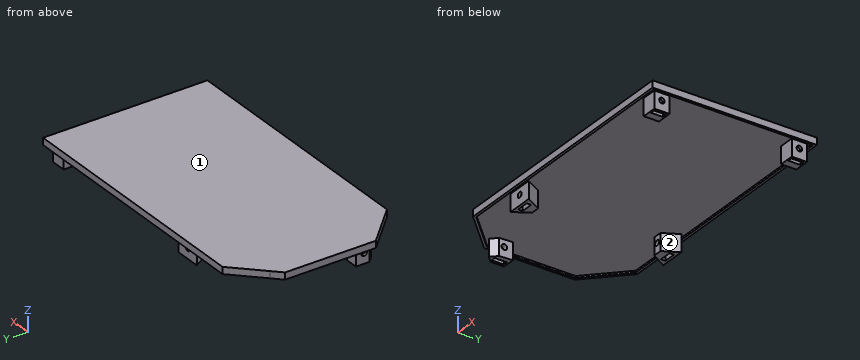
```python
from build123d import *

# Parameters (mm, degrees)
F0_W      = 7.8739928325
F0_H      = 7.8739928325
F1_DEPTH  = 2.54
F2_DEPTH  = 1.016
F3_DEPTH  = 8.89
F8_W      = 2.286
F8_H      = 6.35
F7_W      = 2.286
F7_H      = 6.35
F4_W      = 6.35
F4_H      = 2.286
F5_W      = 2.286
F5_H      = 6.35
F6_W      = 6.35
F6_H      = 2.286
F9_DEPTH  = 8.255
F10_R     = 1.4224
F11_DEPTH = 101.6
F12_R     = 1.4224
F13_R     = 1.4224
F14_DEPTH = 25.4
F15_R     = 1.4224
F16_DEPTH = 25.4


# Not quite as in the source:
# - a feature names something its author has since deleted; it is built from what else it names


with BuildPart() as f1:
    # F0 (on Top) → F1 (new body)
    with BuildSketch(Plane.XY):
        Polygon((-50.5911594971, 45.1345390935), (-65.0638575705, 30.6618410202), (-69.6408525109, 26.0848460797), (-69.6408525109, 9.5127671957), (-69.6408525109, -20.9057678927), (-62.6880467633, -27.8585736403), (-50.5911594971, -39.9554609065), (82.7588405029, -39.9554609065), (82.7588405029, -17.0967224985), (82.7588405029, 43.8645390935), (82.7588405029, 45.1345390935), (33.1444106996, 45.1345390935), (-20.2568043023, 45.1345390935), align=None)
        Polygon((-50.0651082729, -38.6854609065), (-68.3711594971, -20.3794096823), (-68.3711594971, 25.5584878693), (-64.1658319583, 29.763815408), (-50.0651082729, 43.8645390935), (81.4888405029, 43.8645390935), (81.4888405029, -38.6854609065), align=None, mode=Mode.SUBTRACT)
        Polygon((-68.3711594971, 25.5584878693), (-68.3711594971, -20.3794096823), (-50.0651082729, -38.6854609065), (81.4888405029, -38.6854609065), (81.4888405029, 43.8645390935), (-50.0651082729, 43.8645390935), (-64.1658319583, 29.763815408), align=None)
        Polygon((-13.562855112, -36.9074608927), (-27.0518330949, -36.9074608927), (-22.3274411258, -29.0334609202), (-17.8373202542, -29.0334609202), align=None, mode=Mode.SUBTRACT)
        Polygon((-66.5931594971, -19.6429379684), (-66.5931594971, -12.7413552397), (-60.0190392027, -12.7413552397), (-60.413067775, -19.6310556945), (-63.509054773, -22.7270426925), align=None, mode=Mode.SUBTRACT)
        with BuildLine():
            Line((-49.5390570487, -37.4154609065), (-61.7130058245, -25.2415121307))
            Line((-61.7130058245, -25.2415121307), (-58.120903376, -21.6494096823))
            Line((-58.120903376, -21.6494096823), (-56.9411594971, -12.2333584581))
            Line((-56.9411594971, -12.2333584581), (-56.9411594971, -9.6933584581))
            Line((-56.9411594971, -9.6933584581), (-67.1011594971, -9.6933584581))
            Line((-67.1011594971, -9.6933584581), (-67.1011594971, 25.0324366451))
            Line((-67.1011594971, 25.0324366451), (-49.5390570487, 42.5945390935))
            Line((-49.5390570487, 42.5945390935), (-33.3653066841, 42.5945390935))
            ThreePointArc((-33.3653066841, 42.5945390935), (-30.8623950498, 41.9351536832), (-29.0092406655, 40.128174271))
            Line((-29.0092406655, 40.128174271), (-25.1550660971, 33.7045390935))
            ThreePointArc((-25.1550660971, 33.7045390935), (-23.284234992, 31.8649136199), (-20.7556570459, 31.1645390935))
            Line((-20.7556570459, 31.1645390935), (-19.3944751483, 31.1645390935))
            ThreePointArc((-19.3944751483, 31.1645390935), (-16.8544751483, 31.8451300423), (-14.9950660971, 33.7045390935))
            Line((-14.9950660971, 33.7045390935), (-11.6110890868, 39.9381692669))
            ThreePointArc((-11.6110890868, 39.9381692669), (-9.7440488814, 41.8802258253), (-7.1465155593, 42.5945390935))
            Line((-7.1465155593, 42.5945390935), (67.5188405029, 42.5945390935))
            ThreePointArc((67.5188405029, 42.5945390935), (69.3148917271, 41.8505903177), (70.0588405029, 40.0545390935))
            Line((70.0588405029, 40.0545390935), (70.0588405029, 32.4345390935))
            Line((70.0588405029, 32.4345390935), (77.6788405029, 32.4345390935))
            ThreePointArc((77.6788405029, 32.4345390935), (79.4748917271, 31.6905903177), (80.2188405029, 29.8945390935))
            Line((80.2188405029, 29.8945390935), (80.2188405029, -24.7154609065))
            ThreePointArc((80.2188405029, -24.7154609065), (79.4748917271, -26.5115121307), (77.6788405029, -27.2554609065))
            Line((77.6788405029, -27.2554609065), (70.0588405029, -27.2554609065))
            Line((70.0588405029, -27.2554609065), (70.0588405029, -34.8754609065))
            ThreePointArc((70.0588405029, -34.8754609065), (69.3148917271, -36.6715121307), (67.5188405029, -37.4154609065))
            Line((67.5188405029, -37.4154609065), (-7.1465155593, -37.4154609065))
            ThreePointArc((-7.1465155593, -37.4154609065), (-9.7440488814, -36.7011476383), (-11.6110890868, -34.7590910799))
            Line((-11.6110890868, -34.7590910799), (-14.9950660971, -28.5254609065))
            ThreePointArc((-14.9950660971, -28.5254609065), (-16.8544751483, -26.6660518553), (-19.3944751483, -25.9854609065))
            Line((-19.3944751483, -25.9854609065), (-20.7556570459, -25.9854609065))
            ThreePointArc((-20.7556570459, -25.9854609065), (-23.284234992, -26.6858354329), (-25.1550660971, -28.5254609065))
            Line((-25.1550660971, -28.5254609065), (-29.0092406655, -34.949096084))
            ThreePointArc((-29.0092406655, -34.949096084), (-30.8623950498, -36.7560754962), (-33.3653066841, -37.4154609065))
            Line((-33.3653066841, -37.4154609065), (-49.5390570487, -37.4154609065))
        make_face(mode=Mode.SUBTRACT)
        with Locations((75.7738405029, -32.9704609065)):
            Rectangle(F0_W, F0_H, mode=Mode.SUBTRACT)
        Polygon((-27.0518310596, 42.0865379274), (-13.5628570488, 42.0865379274), (-17.8373209399, 34.2125402596), (-22.3274404733, 34.2125402596), align=None, mode=Mode.SUBTRACT)
        with Locations((75.7738405029, 38.1495390935)):
            Rectangle(F0_W, F0_H, mode=Mode.SUBTRACT)
        with BuildLine():
            Line((-58.120903376, -21.6494096823), (-61.7130058245, -25.2415121307))
            Line((-61.7130058245, -25.2415121307), (-49.5390570487, -37.4154609065))
            Line((-49.5390570487, -37.4154609065), (-33.3653066841, -37.4154609065))
            ThreePointArc((-33.3653066841, -37.4154609065), (-30.8623950498, -36.7560754962), (-29.0092406655, -34.949096084))
            Line((-29.0092406655, -34.949096084), (-25.1550660971, -28.5254609065))
            ThreePointArc((-25.1550660971, -28.5254609065), (-23.284234992, -26.6858354329), (-20.7556570459, -25.9854609065))
            Line((-20.7556570459, -25.9854609065), (-19.3944751483, -25.9854609065))
            ThreePointArc((-19.3944751483, -25.9854609065), (-16.8544751483, -26.6660518553), (-14.9950660971, -28.5254609065))
            Line((-14.9950660971, -28.5254609065), (-11.6110890868, -34.7590910799))
            ThreePointArc((-11.6110890868, -34.7590910799), (-9.7440488814, -36.7011476383), (-7.1465155593, -37.4154609065))
            Line((-7.1465155593, -37.4154609065), (67.5188405029, -37.4154609065))
            ThreePointArc((67.5188405029, -37.4154609065), (69.3148917271, -36.6715121307), (70.0588405029, -34.8754609065))
            Line((70.0588405029, -34.8754609065), (70.0588405029, -27.2554609065))
            Line((70.0588405029, -27.2554609065), (77.6788405029, -27.2554609065))
            ThreePointArc((77.6788405029, -27.2554609065), (79.4748917271, -26.5115121307), (80.2188405029, -24.7154609065))
            Line((80.2188405029, -24.7154609065), (80.2188405029, 29.8945390935))
            ThreePointArc((80.2188405029, 29.8945390935), (79.4748917271, 31.6905903177), (77.6788405029, 32.4345390935))
            Line((77.6788405029, 32.4345390935), (70.0588405029, 32.4345390935))
            Line((70.0588405029, 32.4345390935), (70.0588405029, 40.0545390935))
            ThreePointArc((70.0588405029, 40.0545390935), (69.3148917271, 41.8505903177), (67.5188405029, 42.5945390935))
            Line((67.5188405029, 42.5945390935), (-7.1465155593, 42.5945390935))
            ThreePointArc((-7.1465155593, 42.5945390935), (-9.7440488814, 41.8802258253), (-11.6110890868, 39.9381692669))
            Line((-11.6110890868, 39.9381692669), (-14.9950660971, 33.7045390935))
            ThreePointArc((-14.9950660971, 33.7045390935), (-16.8544751483, 31.8451300423), (-19.3944751483, 31.1645390935))
            Line((-19.3944751483, 31.1645390935), (-20.7556570459, 31.1645390935))
            ThreePointArc((-20.7556570459, 31.1645390935), (-23.284234992, 31.8649136199), (-25.1550660971, 33.7045390935))
            Line((-25.1550660971, 33.7045390935), (-29.0092406655, 40.128174271))
            ThreePointArc((-29.0092406655, 40.128174271), (-30.8623950498, 41.9351536832), (-33.3653066841, 42.5945390935))
            Line((-33.3653066841, 42.5945390935), (-49.5390570487, 42.5945390935))
            Line((-49.5390570487, 42.5945390935), (-67.1011594971, 25.0324366451))
            Line((-67.1011594971, 25.0324366451), (-67.1011594971, -9.6933584581))
            Line((-67.1011594971, -9.6933584581), (-56.9411594971, -9.6933584581))
            Line((-56.9411594971, -9.6933584581), (-56.9411594971, -12.2333584581))
            Line((-56.9411594971, -12.2333584581), (-58.120903376, -21.6494096823))
        make_face()
        Polygon((-22.3274411258, -29.0334609202), (-27.0518330949, -36.9074608927), (-13.562855112, -36.9074608927), (-17.8373202542, -29.0334609202), align=None)
        Polygon((-17.8373209399, 34.2125402596), (-13.5628570488, 42.0865379274), (-27.0518310596, 42.0865379274), (-22.3274404733, 34.2125402596), align=None)
        with Locations((75.7738405029, -32.9704609065)):
            Rectangle(F0_W, F0_H)
        with Locations((75.7738405029, 38.1495390935)):
            Rectangle(F0_W, F0_H)
        Polygon((-60.0190392027, -12.7413552397), (-66.5931594971, -12.7413552397), (-66.5931594971, -19.6429379684), (-63.509054773, -22.7270426925), (-60.413067775, -19.6310556945), align=None)
    extrude(amount=F1_DEPTH)

    # F0 (on Top) → F2 (join)
    with BuildSketch(Plane.XY):
        Polygon((-50.5911594971, 45.1345390935), (-65.0638575705, 30.6618410202), (-69.6408525109, 26.0848460797), (-69.6408525109, 9.5127671957), (-69.6408525109, -20.9057678927), (-62.6880467633, -27.8585736403), (-50.5911594971, -39.9554609065), (82.7588405029, -39.9554609065), (82.7588405029, -17.0967224985), (82.7588405029, 43.8645390935), (82.7588405029, 45.1345390935), (33.1444106996, 45.1345390935), (-20.2568043023, 45.1345390935), align=None)
        Polygon((-50.0651082729, -38.6854609065), (-68.3711594971, -20.3794096823), (-68.3711594971, 25.5584878693), (-64.1658319583, 29.763815408), (-50.0651082729, 43.8645390935), (81.4888405029, 43.8645390935), (81.4888405029, -38.6854609065), align=None, mode=Mode.SUBTRACT)
    extrude(amount=-F2_DEPTH)

    # F0 (on Top) → F3 (join)
    with BuildSketch(Plane.XY):
        Polygon((-17.8373209399, 34.2125402596), (-13.5628570488, 42.0865379274), (-27.0518310596, 42.0865379274), (-22.3274404733, 34.2125402596), align=None)
        Polygon((-22.3274411258, -29.0334609202), (-27.0518330949, -36.9074608927), (-13.562855112, -36.9074608927), (-17.8373202542, -29.0334609202), align=None)
        Polygon((-60.0190392027, -12.7413552397), (-66.5931594971, -12.7413552397), (-66.5931594971, -19.6429379684), (-63.509054773, -22.7270426925), (-60.413067775, -19.6310556945), align=None)
        with Locations((75.7738405029, -32.9704609065)):
            Rectangle(F0_W, F0_H)
        with Locations((75.7738405029, 38.1495390935)):
            Rectangle(F0_W, F0_H)
    extrude(amount=-F3_DEPTH)

    # F8 (on face) + F7 (on face) + F4 (on face) + F5 (on face) + F6 (on face) → F9 (cut)
    with BuildSketch(Plane(origin=(0, 0, -8.89), x_dir=(1, 0, 0), z_dir=(0, 0, -1))):
        with Locations((77.1708369192, -38.1495390935)):
            Rectangle(F8_W, F8_H)
    with BuildSketch(Plane(origin=(0, 0, -8.89), x_dir=(1, 0, 0), z_dir=(0, 0, -1))):
        with Locations((77.1708369192, 32.9704609065)):
            Rectangle(F7_W, F7_H)
    with BuildSketch(Plane(origin=(0, 0, -8.89), x_dir=(1, 0, 0), z_dir=(0, 0, -1))):
        with Locations((-20.3073441034, 34.3674608927)):
            Rectangle(F4_W, F4_H)
    with BuildSketch(Plane(origin=(0, 0, -8.89), x_dir=(1, 0, 0), z_dir=(0, 0, -1))):
        with Locations((-64.0531594971, 16.9871170074)):
            Rectangle(F5_W, F5_H)
    with BuildSketch(Plane(origin=(0, 0, -8.89), x_dir=(1, 0, 0), z_dir=(0, 0, -1))):
        with Locations((-20.3073440542, -39.5465379274)):
            Rectangle(F6_W, F6_H)
    extrude(amount=-F9_DEPTH, mode=Mode.SUBTRACT)

    # F10 (on face) → F11 (cut)
    with BuildSketch(Plane(origin=(0, 42.0865379274, 0), x_dir=(-1, 0, 0), z_dir=(0, 1, 0))):
        with Locations((20.3073440542, -3.683)):
            Circle(F10_R)
    extrude(amount=-F11_DEPTH, mode=Mode.SUBTRACT)

    # F12 (on face) + F13 (on face) → F14 (cut)
    with BuildSketch(Plane.YZ.offset(79.7108369192)):
        with Locations((38.1495390935, -3.683)):
            Circle(F12_R)
    with BuildSketch(Plane.YZ.offset(79.7108369192)):
        with Locations((-32.9704609065, -3.683)):
            Circle(F13_R)
    extrude(amount=-F14_DEPTH, mode=Mode.SUBTRACT)

    # F15 (on face) → F16 (cut)
    with BuildSketch(Plane(origin=(-66.5931594971, 0, 0), x_dir=(0, -1, 0), z_dir=(-1, 0, 0))):
        with Locations((16.9831552397, -3.683)):
            Circle(F15_R)
    extrude(amount=-F16_DEPTH, mode=Mode.SUBTRACT)


solid = f1.part
```
For this review, take the finished solid that the model builds, in its own axes (mm). Face numbers are marked on the shaded views. Coordinates: 2 decimals unless noted, no trailing zeros. Write each loop counter-clockwise with the first axis right and the second up, starting at its lowest first coordinate (ties: lowest second). Pieces come first, ordered by that corner, then holes. Notation, with made-up numbers: (20, 69.25) - (33, 69.25) arc R24 cw to (33, 89.25) - close; hole circle Ø11 at (73.5, 33). An arc over 180 degrees is marked (long way). Put each result on its own line as item: value.
1. Add section B-B, the plane x = 1.5. Give the boundary of the cut face in (y, z), then the cut area to 3 significant figures.
Values found:
outline: (-39.96, -1.02) - (-38.69, -1.02) - (-38.69, 0) - (43.86, 0) - (43.86, -1.02) - (45.13, -1.02) - (45.13, 2.54) - (-39.96, 2.54) - close
area: 219 mm²
2. Add section A-A, the plane z = -6.75. Count the separate pieces of the cut face and the enclosed holes in it, then the cut area to 3 significant figures.
Values found:
separate pieces: 5
enclosed holes: 5
area: 247 mm²
3. Add section C-C, the plane y = -17. Give the boundary of the cut face in (x, z) (3 decimals), then the cut area to 3 significant figures.
Values found:
outline: (-69.641, -1.016) - (-68.371, -1.016) - (-68.371, 0) - (-66.593, 0) - (-66.593, -2.261) - (-65.196, -2.261) - (-65.196, -0.635) - (-62.91, -0.635) - (-62.91, -2.261) - (-60.263, -2.261) - (-60.263, 0) - (81.489, 0) - (81.489, -1.016) - (82.759, -1.016) - (82.759, 2.54) - (-69.641, 2.54) - close; (-66.593, -8.89) - (-65.196, -8.89) - (-65.196, -5.105) - (-66.593, -5.105) - close; (-62.91, -8.89) - (-60.263, -8.89) - (-60.263, -5.105) - (-62.91, -5.105) - close
area: 416 mm²
4. Mouldability with a two-part tool opening along X and no side actions: class the marked faces 1 and 2 as released by +X, released by -X, zero draft, split by the parting line, or undercut.
Values found:
face 1: zero draft
face 2: undercut
5. Add section D-D, the plane y = 24. Give the boundary of the cut face in (x, z), then the cut area to 3 significant figures.
Values found:
outline: (-69.64, -1.02) - (-68.37, -1.02) - (-68.37, 0) - (81.49, 0) - (81.49, -1.02) - (82.76, -1.02) - (82.76, 2.54) - (-69.64, 2.54) - close
area: 390 mm²
6. For pin 1 (1 mm diameter, centred on x = -28.5, y = 19, fed in from -Z); pin 2 (3.5 mm diameter, centred on y = -16.98, z = -3.68, fed in from +X); pin 3 (2.5 mm diameter, centred on y = 38, z = -6.5, fed in from +X), all flat-tipped, find the tip position at first contact; note any pin that passes through.
Values found:
pin 1: z = 0
pin 2: x = -60.16
pin 3: x = 79.71
7. Wall thickness on probe 1 along X at (y, z) = (-30, -2.5); probe 2 along Z at (x, y) = (30.5, -19.5); probe 3 along X at (y, z) = (41, -7.5): over which ranges is each line inside the solid? List them lowest first.
Values found:
probe 1: -22.91 to -21.1, -19.52 to -17.31, 71.84 to 76.03, 78.31 to 79.71
probe 2: 0 to 2.54
probe 3: -26.4 to -14.15, 71.84 to 76.03, 78.31 to 79.71
